Print and shaded views of the part. All mm, measured from the part's lowest x, y and z. A direction names the side the tool comes from. Give positions to 0.01 mm unless a question says otherwise; leave off trailing zeros. Order: outer loops, then holes, each group sorted by start corner. A loop starts at its lowest first (then second) coordinate and runs counter-clockwise, first axis right, second up. Notation, with made-up numbers: (27, 66.25) -> (65, 66.25) arc R17 ccw to (65, 96.25) -> close; hole circle Ø3 at (47.5, -26.5). An arc over 180 degrees is marked (long way). One line per question, with ' | ' between items. Start each with the question number.
(1) Which spindle directions (+Z, -Z, +X, -X, +Y, -Y) get a long thin tool onto all of the face, cutting with end or side? Do the marked faces 4 and 5. Say none if no direction does.
(2) Pin check, flat tips, straight feed: pin 1 Ø1 at (x, z) = (75, 12.5) entering from +Y; pin 2 Ø0.6 at (x, y) = (17.5, 32) entering from -Z; pin 3 Ø1 at (y, z) = (32.5, 19) entering from -X. Stop position of each tip, or through.
(3) Drill centre lines: L1, parallel to Y at x = 142, z = 21.5; L2, parallel to Y at x = 27.5, z = 26.5; L3, parallel to X at y = 4, z = 8.5 (1 decimal). Where is each one in solid material? Low to high. Write a range as from..to.
(4) Cut at B-B (x = 100). Give the cut face in (y, z).
(5) Cut at C-C (z = 25). Give the cut face in (x, y) (1 decimal).
(6) Cut at A-A (z = 33.5). Give the cut face in (x, y) (1 decimal), then the cut area to 3 significant figures.
(7) Cut at D-D (y = 6.5). Give the cut face in (x, z) (1 decimal), then the cut area to 3 significant figures.
(8) Pull direction X, two halves, no side cores. Call the marked faces 1, 2 and 3: +X half, -X half, draft (parallel to the pull), parting line (faces both ways), or undercut.
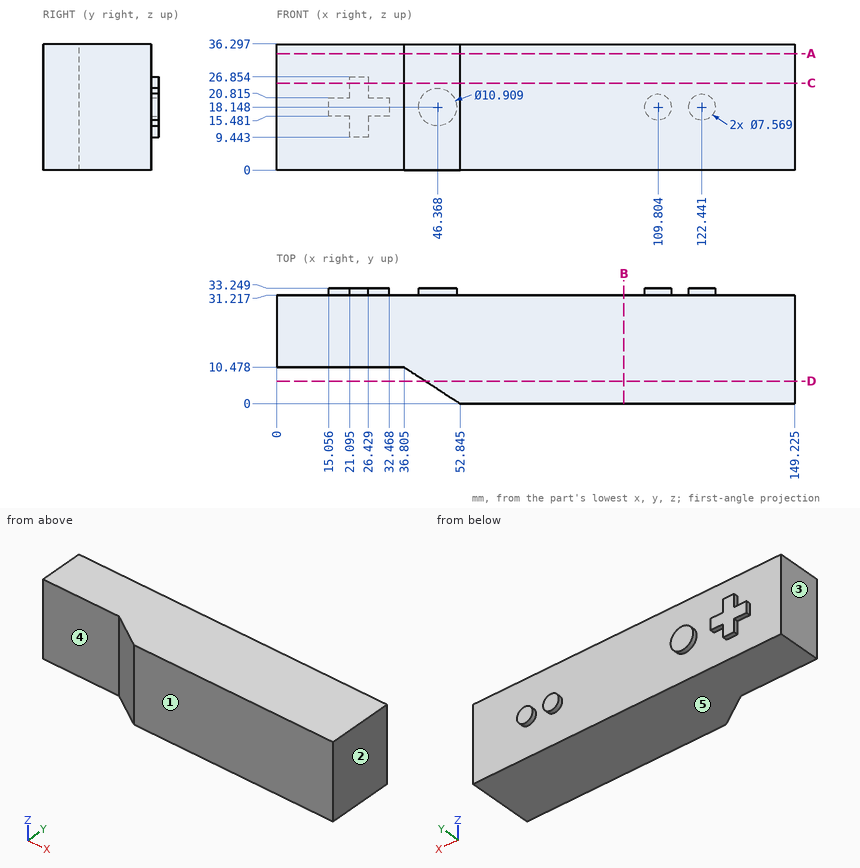
Result set:
1) face 4: +Z, -Z, -X, -Y | face 5: -Z, +X, -X, +Y, -Y
2) pin 1: stops at y = 31.22 | pin 2: stops at z = 15.48 | pin 3: stops at x = 15.06
3) L1: y = 0..31.22 | L2: y = 10.48..31.22 | L3: x = 46.7..149.2
4) outline: (0, 0) -> (31.22, 0) -> (31.22, 36.3) -> (0, 36.3) -> close
5) outline: (0, 10.5) -> (36.8, 10.5) -> (52.8, 0) -> (149.2, 0) -> (149.2, 31.2) -> (26.4, 31.2) -> (26.4, 33.2) -> (21.1, 33.2) -> (21.1, 31.2) -> (0, 31.2) -> close
6) outline: (0, 10.5) -> (36.8, 10.5) -> (52.8, 0) -> (149.2, 0) -> (149.2, 31.2) -> (0, 31.2) -> close | area: 4,190 mm2
7) outline: (42.9, 0) -> (149.2, 0) -> (149.2, 36.3) -> (42.9, 36.3) -> close | area: 3,860 mm2
8) face 1: draft | face 2: +X half | face 3: -X half
